Input: part model. Units: mm. Frame: model coordinates. Coordinates: 2 decimals unless noted, no trailing zeros. Order: outer loops, then holes, each group sorted by start corner. A loop starts at its lowest first (then second) coordinate and runs counter-clockwise, first axis right, second up. Notation, with made-up numbers: (-16, 78) -> (4, 78) arc R22 ccw to (4, 99) -> close; hole circle Ø9 at (-30.5, 29). An arc over 180 degrees is marked (long way). One line per item, written item: value. Start each with the question number.
from build123d import *

# Parameters (mm, degrees)
BOSS_EXTRUDE1_DEPTH = 3.175
CUT_EXTRUDE1_DEPTH  = 204.138678001
SKETCH3_W           = 42
SKETCH3_H           = 55.35
SKETCH3_W_2         = 7
SKETCH3_H_2         = 10
SKETCH3_W_3         = 7.65
SKETCH3_H_3         = 6.35
CUT_EXTRUDE2_DEPTH  = 204.138678001
FILLET3_R           = 5
SKETCH4_R           = 2
CUT_EXTRUDE3_DEPTH  = 204.138678001
CUT_EXTRUDE4_DEPTH  = 204.138678001
FILLET4_R           = 76
FILLET5_R           = 7


with BuildPart() as part:
    # Sketch1 → Boss-Extrude1 (new, symmetric)
    with BuildSketch(Plane(origin=(0, 0, 0), x_dir=(1, 0, 0), z_dir=(0, 1, 0))):
        with BuildLine():
            Line((35, -200), (35, 0))
            ThreePointArc((35, 0), (0, 35), (-35, 0))
            Line((-35, 0), (-35, -200))
            Line((-35, -200), (35, -200))
        make_face()
    extrude(amount=BOSS_EXTRUDE1_DEPTH, both=True)

    # Sketch2 → Cut-Extrude1 (cut, through all)
    with BuildSketch(Plane(origin=(0, 3.175, 0), x_dir=(1, 0, 0), z_dir=(0, 1, 0))):
        with BuildLine():
            Line((-35, -38), (35, -38))
            Line((35, -38), (35, 0))
            ThreePointArc((35, 0), (0, 35), (-35, 0))
            Line((-35, 0), (-35, -38))
        make_face()
    extrude(amount=-CUT_EXTRUDE1_DEPTH, mode=Mode.SUBTRACT)

    # Sketch3 → Cut-Extrude2 (cut, through all)
    with BuildSketch(Plane(origin=(0, 3.175, 0), x_dir=(1, 0, 0), z_dir=(0, 1, 0))):
        with Locations((0, -162.325)):
            Rectangle(SKETCH3_W, SKETCH3_H)
        with Locations((0, -195)):
            Rectangle(SKETCH3_W_2, SKETCH3_H_2)
        with Locations((-24.825, -186.825)):
            Rectangle(SKETCH3_W_3, SKETCH3_H_3)
        with Locations((24.825, -186.825)):
            Rectangle(SKETCH3_W_3, SKETCH3_H_3)
    extrude(amount=-CUT_EXTRUDE2_DEPTH, mode=Mode.SUBTRACT)

    # Fillet3
    fillet3_edges = [part.edges().sort_by_distance(p)[0] for p in [
        (3.5, 0, 200),
        (-3.5, 0, 200),
        (35, 0, 200),
        (-35, 0, 200),
    ]]
    fillet(fillet3_edges, radius=FILLET3_R)

    # Sketch4 → Cut-Extrude3 (cut, through all)
    with BuildSketch(Plane(origin=(0, 3.175, 0), x_dir=(1, 0, 0), z_dir=(0, 1, 0))):
        with Locations(Location((15, -65.35, 0), (0, 0, 270))):
            Circle(SKETCH4_R)
        with Locations(Location((-15, -65.35, 0), (0, 0, 270))):
            Circle(SKETCH4_R)
        with Locations(Location((27.5, -195.35, 0), (0, 0, 270))):
            Circle(SKETCH4_R)
        with Locations(Location((-27.5, -195.35, 0), (0, 0, 270))):
            Circle(SKETCH4_R)
    extrude(amount=-CUT_EXTRUDE3_DEPTH, mode=Mode.SUBTRACT)

    # Sketch5 → Cut-Extrude4 (cut, through all)
    with BuildSketch(Plane(origin=(0, 3.175, 0), x_dir=(1, 0, 0), z_dir=(0, 1, 0))):
        with BuildLine():
            Line((-35, -134.65), (-35, -49.65))
            ThreePointArc((-35, -49.65), (-18.102907984, -92.15), (-35, -134.65))
        make_face()
    cut_extrude4 = extrude(amount=-CUT_EXTRUDE4_DEPTH, mode=Mode.SUBTRACT)

    # Mirror1: Cut-Extrude4 across plane
    add(cut_extrude4.mirror(Plane(origin=(0, 0, 0), x_dir=(0, 0, 1), z_dir=(1, 0, 0))), mode=Mode.SUBTRACT)

    # Fillet4
    # the kernel refuses this fillet: 76 mm, written as the material it takes off along each edge
    with BuildSketch(Plane(origin=(-35, 39.601520625, 49.65), x_dir=(0, 0, -1), z_dir=(0, -1, 0))) as fillet4_piece_1:
        with BuildLine():
            CenterArc((26.124451555, 74.608915367), FILLET4_R, 240.155370723, 18.865389254)
            Line((-11.696928446, 8.688181035), (-12.453356046, 7.369766348))
            ThreePointArc((-12.453356046, 7.369766348), (-6.498269887, 3.469254885), (-1.04366777, -1.105059992))
            Line((-1.04366777, -1.105059992), (0, -1.52))
            ThreePointArc((0, -1.52), (5.825, -1.52), (11.360510969, -1.492178307))
            Line((11.360510969, -1.492178307), (11.65, 0))
        make_face()
    extrude(amount=79.20304125, mode=Mode.SUBTRACT)
    with BuildSketch(Plane(origin=(-35, 62.277048415, 134.65), x_dir=(0.587963491001448, 0, -0.8088874663693276), z_dir=(0, -1, 0))) as fillet4_piece_2:
        with BuildLine():
            CenterArc((25.562462836, 75.375386129), FILLET4_R, 233.987375861, 28.66182532)
            Line((-19.12276248, 13.899938684), (-20.016466986, 12.670429736))
            Line((-20.016466986, 12.670429736), (-0.893704506, -1.229508949))
            Line((-0.893704506, -1.229508949), (0.194474848, -1.507507723))
            ThreePointArc((0.194474848, -1.507507723), (7.919360226, -1.011292338), (15.644245604, -1.507507723))
            Line((15.644245604, -1.507507723), (15.838720451, 0))
        make_face()
    extrude(amount=124.554096829, mode=Mode.SUBTRACT)
    with BuildSketch(Plane(origin=(35, 62.277048415, 134.65), x_dir=(-0.587963491001448, 0, -0.8088874663693276), z_dir=(0, -1, 0))) as fillet4_piece_3:
        with BuildLine():
            CenterArc((25.562462836, -75.375386129), FILLET4_R, 97.350798819, 28.66182532)
            Line((-19.12276248, -13.899938684), (-20.016466986, -12.670429736))
            Line((-20.016466986, -12.670429736), (-0.893704506, 1.229508949))
            Line((-0.893704506, 1.229508949), (0.194474848, 1.507507723))
            ThreePointArc((0.194474848, 1.507507723), (7.919360226, 1.011292338), (15.644245604, 1.507507723))
            Line((15.644245604, 1.507507723), (15.838720451, 0))
        make_face()
    extrude(amount=124.554096829, mode=Mode.SUBTRACT)
    with BuildSketch(Plane(origin=(35, 39.601520625, 49.65), x_dir=(0, 0, -1), z_dir=(0, -1, 0))) as fillet4_piece_4:
        with BuildLine():
            CenterArc((26.124451555, -74.608915367), FILLET4_R, 100.979240023, 18.865389254)
            Line((-11.696928446, -8.688181035), (-12.453356046, -7.369766348))
            ThreePointArc((-12.453356046, -7.369766348), (-6.498269887, -3.469254885), (-1.04366777, 1.105059992))
            Line((-1.04366777, 1.105059992), (0, 1.52))
            ThreePointArc((0, 1.52), (5.825, 1.52), (11.360510969, 1.492178307))
            Line((11.360510969, 1.492178307), (11.65, 0))
        make_face()
    extrude(amount=79.20304125, mode=Mode.SUBTRACT)

    # Fillet5
    fillet5_edges = [part.edges().sort_by_distance(p)[0] for p in [
        (35, 0, 38),
        (-35, 0, 38),
    ]]
    fillet(fillet5_edges, radius=FILLET5_R)


solid = part.part
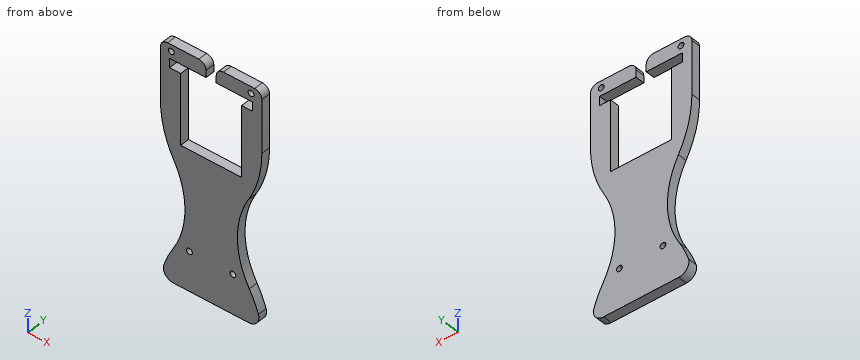
1) Section query A-A, the plane x = 15. Return the cut outline in (y, z) (3 decimals), plus the area to 3 significant figures.
2) Section query D-D, the plane x = 22.5. Return the cut outline in (y, z) (3 decimals).
3) Section query C-C, the plane z = 148. Return the cut outline in (x, y) (3 decimals), plus the area to 3 significant figures.
4) Section query B-B, the plane y = 0. State how many separate pieces and enclosed holes the cut face has, plus the area to 3 significant figures.
5) Pin query (flat end, axial travel): pin 1 Ø3.5 at (x, z) = (-15, 65.35) entering from -Y; pin 2 Ø1.5 at (y, z) = (2, 108) entering from -X. Return the tip coordinate at first contact, or that it passes through.
6) Ray query, line 1 along X through (y, z) = (1.25, 195.35); line 2 along X through (y, z) = (-1.25, 179); line 3 along Z through (x, y) = (16, 2.75). Return the intervals inside material, ascending. Write a range as from..to.
Entries:
1. outline: (-3.175, 38) -> (3.175, 38) -> (3.175, 63.35) -> (-3.175, 63.35) -> close; (-3.175, 67.35) -> (3.175, 67.35) -> (3.175, 134.65) -> (-3.175, 134.65) -> close; (-3.175, 190) -> (3.175, 190) -> (3.175, 200) -> (-3.175, 200) -> close
1. area: 652 mm2
2. outline: (-3.175, 38) -> (3.175, 38) -> (3.175, 69.237) -> (-3.175, 69.237) -> close; (-3.175, 115.063) -> (3.175, 115.063) -> (3.175, 183.65) -> (-3.175, 183.65) -> close; (-3.175, 190) -> (3.175, 190) -> (3.175, 200) -> (-3.175, 200) -> close
3. outline: (-34.3, -3.175) -> (-21, -3.175) -> (-21, 3.175) -> (-34.3, 3.175) -> close; (21, -3.175) -> (34.3, -3.175) -> (34.3, 3.175) -> (21, 3.175) -> close
3. area: 169 mm2
4. separate pieces: 1
4. enclosed holes: 4
4. area: 6,610 mm2
5. pin 1: passes through
5. pin 2: stops at x = -20.37
6. line 1: x = -34.99..-29.5, -25.5..-3.51, 3.51..25.5, 29.5..34.99
6. line 2: x = -35..-21, 21..35
6. line 3: z = 38..63.62, 67.08..134.65, 190..200
